Check sheet for the modelled part. Datum: model origin and axes. Units: mm. A direction names the side the tool comes from. Round coordinates to 2 decimals unless told otherwise and drop trailing zeros. Order: outer loops, then holes, each group sorted by start corner. A loop starts at its lowest first (then second) coordinate and runs counter-clockwise, first axis right, second up. Notation, with made-up numbers: (66, 0.5) -> (78, 0.5) arc R23 ccw to (78, 10.5) -> close; hole circle Ø3 at (79, 27.5). An arc over 180 degrees is marked (long way). Answer in a Markdown table with one row per item. Add a question column.
1. Sectioned sample at B-B, the plane z = 25. Record the boundary of the cut face in (x, y), then the cut area to 3 significant figures.
2. Sectioned sample at A-A, the plane x = 1. Record the boundary of the cut face in (y, z).
3. Draft check along Z on faces 1 (the flat face through (20, 0, 0)), 2 (the flat face through (-20, 0, -20)), 3 (the flat face through (-11, -11, 35)). Enter one of: +Z half, -Z half, draft (parallel to the pull), parting line (faces both ways), or undercut.
4. Access from +Z, -Z, +X, -X, +Y, -Y to the whole of each face (thin tool, end or side, straight path). Record for faces 4 (the flat face through (0, 0, 5)), 5 (the cylindrical face through (-19, 0, -7)), 6 (the flat face through (18, 18, 5)), 7 (the flat face through (-18, -18, 5)), 8 (the flat face through (18, -18, 5)).
5. Sectioned sample at C-C, the plane y = -1. Record the boundary of the cut face in (x, z), then the cut area to 3 significant figures.
6. Depth check by flat-ended pin: P1, Ø16, axis at y = 4, z = -24.5, coming from the +X side; P2, Ø6, axis at y = 14, z = -27.5, coming from the +X side; P3, Ø3, axis at x = -15.5, z = 24.5, coming from the -Y side. Enter the tip coordinate at first touch or a pass-through.
7. Material ranges on L1, parallel to Z at x = 11, y = -5.5; L2, parallel to Z at x = -2.5, y = 16; L3, parallel to Y at x = 6, z = 14, recorded low to high. Write a range as from..to.
8. Sectioned sample at D-D, the plane z = -6. Record the boundary of the cut face in (x, y).
```python
from build123d import *

# Parameters (mm, degrees)
F1_DEPTH = 20
F3_DEPTH = 30


# Not quite as in the source:
# - a fillet or chamfer that OpenCascade refuses, or shapes differently, is made with other operations: its cross-section is extruded or revolved along the edge and cut away or added
# - a feature names something its author has since deleted; it is built from what else it names


with BuildPart() as f1:
    # F0 (on Front) → F1 (new body, symmetric)
    with BuildSketch(Plane.XZ):
        with BuildLine():
            Line((-10, -5), (20, -5))
            Line((20, -5), (20, 5))
            Line((20, 5), (-20, 5))
            ThreePointArc((-20, 5), (-27.0710678119, 2.0710678119), (-30, -5))
            Line((-30, -5), (-30, -37.0084848255))
            Line((-30, -37.0084848255), (-29.9999700785, -37.1900333921))
            ThreePointArc((-29.9999700785, -37.1900333921), (-27.134358967, -44.1955599538), (-20.1815186475, -47.1867371371))
            Line((-20.1815186475, -47.1867371371), (-20, -47.1900331229))
            Line((-20, -47.1900331229), (20, -47.1900331229))
            Line((20, -47.1900331229), (20, -35))
            Line((20, -35), (-15, -35))
            ThreePointArc((-15, -35), (-18.5355339059, -33.5355339059), (-20, -30))
            Line((-20, -30), (-20, -15))
            Line((-20, -15), (-20, -10))
            ThreePointArc((-20, -10), (-18.5355339059, -6.4644660941), (-15, -5))
            Line((-15, -5), (-10, -5))
        make_face()
    extrude(amount=F1_DEPTH, both=True)

    # F2 (on face) → F3 (join)
    with BuildSketch(Plane.XY.offset(5)):
        with BuildLine():
            Line((-11, 11), (-2, 11))
            ThreePointArc((-2, 11), (-4.6360389693, 17.3639610307), (-11, 20))
            Line((-11, 20), (-11, 11))
        make_face()
        with BuildLine():
            Line((-20, 11), (-11, 11))
            Line((-11, 11), (-11, 20))
            ThreePointArc((-11, 20), (-17.3639610307, 17.3639610307), (-20, 11))
        make_face()
        with BuildLine():
            ThreePointArc((-20, 11), (-17.3639610288, 4.6360389675), (-10.9999999948, 2))
            Line((-11, 2), (-11, 11))
            Line((-11, 11), (-20, 11))
        make_face()
        with BuildLine():
            Line((-11, 11), (-11, 2))
            ThreePointArc((-10.9999999948, 2), (-4.6360389675, 4.6360389712), (-2, 11))
            Line((-2, 11), (-11, 11))
        make_face()
        with BuildLine():
            ThreePointArc((11, 20), (4.6360389693, 17.3639610307), (2, 11))
            Line((2, 11), (11, 11))
            Line((11, 11), (11, 20))
        make_face()
        with BuildLine():
            Line((11, 20), (11, 11))
            Line((11, 11), (20, 11))
            ThreePointArc((20, 11), (17.3639610307, 17.3639610307), (11, 20))
        make_face()
        with BuildLine():
            Line((11, 11), (11, 2))
            ThreePointArc((11, 2), (17.3639610307, 4.6360389693), (20, 11))
            Line((20, 11), (11, 11))
        make_face()
        with BuildLine():
            ThreePointArc((2, 11), (4.6360389693, 4.6360389693), (11, 2))
            Line((11, 2), (11, 11))
            Line((11, 11), (2, 11))
        make_face()
        with BuildLine():
            ThreePointArc((11, -2), (4.6360389693, -4.6360389693), (2, -11))
            Line((2, -11), (11, -11))
            Line((11, -11), (11, -2))
        make_face()
        with BuildLine():
            Line((11, -2), (11, -11))
            Line((11, -11), (20, -11))
            ThreePointArc((20, -11), (17.3639610307, -4.6360389693), (11, -2))
        make_face()
        with BuildLine():
            Line((11, -11), (11, -20))
            ThreePointArc((11, -20), (17.3639610307, -17.3639610307), (20, -11))
            Line((20, -11), (11, -11))
        make_face()
        with BuildLine():
            Line((11, -11), (2, -11))
            ThreePointArc((2, -11), (4.6360389693, -17.3639610307), (11, -20))
            Line((11, -20), (11, -11))
        make_face()
        with BuildLine():
            ThreePointArc((-11, -20), (-4.6360389693, -17.3639610307), (-2, -11))
            Line((-2, -11), (-11, -11))
            Line((-11, -11), (-11, -20))
        make_face()
        with BuildLine():
            ThreePointArc((-20, -11), (-17.3639610307, -17.3639610307), (-11, -20))
            Line((-11, -20), (-11, -11))
            Line((-11, -11), (-20, -11))
        make_face()
        with BuildLine():
            Line((-20, -11), (-11, -11))
            Line((-11, -11), (-11, -2))
            ThreePointArc((-11, -2), (-17.3639610307, -4.6360389693), (-20, -11))
        make_face()
        with BuildLine():
            Line((-11, -11), (-2, -11))
            ThreePointArc((-2, -11), (-4.6360389693, -4.6360389693), (-11, -2))
            Line((-11, -2), (-11, -11))
        make_face()
    extrude(amount=F3_DEPTH)

    # F4: fillet of radius 2.5 on 4 edges, made by hand

    # F4_s1 → F4_t2 (revolve, cut)
    with BuildSketch(Plane.YZ.offset(-11)):
        with BuildLine():
            ThreePointArc((2, 32.5), (2.732233047, 34.267766953), (4.5, 35))
            Line((4.5, 35), (2, 35))
            Line((2, 35), (2, 32.5))
        make_face()
    revolve(axis=Axis((-11, 11, 35), (0, 0, 1)), mode=Mode.SUBTRACT)

    # F4_s3 → F4_t4 (revolve, cut)
    with BuildSketch(Plane.XZ.offset(-11)):
        with BuildLine():
            ThreePointArc((2, 32.5), (2.732233047, 34.267766953), (4.5, 35))
            Line((4.5, 35), (2, 35))
            Line((2, 35), (2, 32.5))
        make_face()
    revolve(axis=Axis((11, 11, 35), (0, 0, 1)), mode=Mode.SUBTRACT)

    # F4_s5 → F4_t6 (revolve, cut)
    with BuildSketch(Plane.XZ.offset(11)):
        with BuildLine():
            ThreePointArc((2, 32.5), (2.732233047, 34.267766953), (4.5, 35))
            Line((4.5, 35), (2, 35))
            Line((2, 35), (2, 32.5))
        make_face()
    revolve(axis=Axis((11, -11, 35), (0, 0, 1)), mode=Mode.SUBTRACT)

    # F4_s7 → F4_t8 (revolve, cut)
    with BuildSketch(Plane.XZ.offset(11)):
        with BuildLine():
            ThreePointArc((-2, 32.5), (-2.732233047, 34.267766953), (-4.5, 35))
            Line((-4.5, 35), (-2, 35))
            Line((-2, 35), (-2, 32.5))
        make_face()
    revolve(axis=Axis((-11, -11, 35), (0, 0, 1)), mode=Mode.SUBTRACT)


solid = f1.part
```
Answer key:
| question | item | result |
|---|---|---|
| 1 | outline | circle Ø18 at (-11, -11); circle Ø18 at (-11, 11); circle Ø18 at (11, -11); circle Ø18 at (11, 11) |
| 1 | area | 1,020 mm² |
| 2 | outline | (-20, -47.19) -> (20, -47.19) -> (20, -35) -> (-20, -35) -> close; (-20, -5) -> (20, -5) -> (20, 5) -> (-20, 5) -> close |
| 3 | face 1 | draft |
| 3 | face 2 | undercut |
| 3 | face 3 | +Z half |
| 4 | face 4 | +Z |
| 4 | face 5 | +X, +Y, -Y |
| 4 | face 6 | +Z, +X, +Y |
| 4 | face 7 | +Z, -X, -Y |
| 4 | face 8 | +Z, +X, -Y |
| 5 | outline | (-30, -37.19) arc R10 ccw to (-20.18, -47.19) -> (-20, -47.19) -> (20, -47.19) -> (20, -35) -> (-15, -35) arc R5 cw to (-20, -30) -> (-20, -10) arc R5 cw to (-15, -5) -> (20, -5) -> (20, 5) -> (-20, 5) arc R10 ccw to (-30, -5) -> (-30, -37.01) -> close |
| 5 | area | 1,380 mm² |
| 6 | P1 | stops at x = -19.33 |
| 6 | P2 | stops at x = -19.97 |
| 6 | P3 | stops at y = -19.49 |
| 7 | L1 | z = -47.19..-35, -5..35 |
| 7 | L2 | z = -47.19..-35, -5..5 |
| 7 | L3 | y = -18.48..-3.52, 3.52..18.48 |
| 8 | outline | (-30, -20) -> (-18, -20) -> (-18, 20) -> (-30, 20) -> close |
